Geometry: final body of the model. Coordinates: model frame, mm. A direction names the side the tool comes from. Coordinates: 2 decimals unless noted, no trailing zeros. Order: outer loops, then holes, each group sorted by start corner. A loop starts at its lowest first (then second) coordinate and runs counter-clockwise, first axis right, second up. Notation, with made-up numbers: (-19.75, -11.75) -> (13.25, -11.75) arc R14 cw to (13.25, 8.25) -> close; hole circle Ø1 at (-18.5, -26.5). An arc over 180 degrees is marked (long way). Answer in a Markdown table with one row per item. Add a question column.
1) Ray query, line 1 (Y direction, x = -302, z = -784); line 2 (Z direction, x = -180, y = -136). Return the intervals inside material, ascending. Write a range as from..to.
2) Contact query for flat-ended pins moving along their axis: P1, Ø1.5, axis at x = -223.5, z = -242, coming from the -Y side; P2, Ø4, axis at y = -2, z = -550, coming from the -X side; P3, Ø2, axis at x = -126.5, z = -216, coming from the +Y side. Output: stop coordinate, or through.
3) Section query C-C on z = -466. Return the cut outline in (x, y).
4) Section query A-A on x = -193.5. Return the cut outline in (y, z).
5) Section query B-B on y = -115. Return the cut outline in (x, z), then the cut area to 3 significant figures.
6) Set-up query: faces 1 (the face through (-218, -5.08, -430)), 2 (the face through (-219, 0, -439)). Return all of +Z, -Z, +X, -X, +Y, -Y with unobstructed straight access to the full face (end or side cutting, diameter ignored); none if empty.
```python
from build123d import *

# Parameters (mm, degrees)
F0_W     = 429.031141
F0_H     = 871.334374
F1_DEPTH = 5.08
F2_W     = 431.302786
F2_H     = 296.81766
F3_DEPTH = 5.08


with BuildPart() as f1:
    # F0 (on Front) → F1 (new body)
    with BuildSketch(Plane.XZ):
        with Locations((-214.51557, -435.667187)):
            Rectangle(F0_W, F0_H)
    extrude(amount=F1_DEPTH)

    # F2 (on Top) → F3 (join)
    with BuildSketch(Plane.XY):
        with Locations((-215.651393, -148.40883)):
            Rectangle(F2_W, F2_H)
    extrude(amount=F3_DEPTH)


solid = f1.part
```
Result:
| question | item | result |
|---|---|---|
| 1 | line 1 | -5.08..0 |
| 1 | line 2 | 0..5.08 |
| 2 | P1 | y = -5.08 |
| 2 | P2 | x = -429.03 |
| 2 | P3 | y = 0 |
| 3 | outline | (-429.03, -5.08) -> (0, -5.08) -> (0, 0) -> (-429.03, 0) -> close |
| 4 | outline | (-296.82, 0) -> (-5.08, 0) -> (-5.08, -871.33) -> (0, -871.33) -> (0, 5.08) -> (-296.82, 5.08) -> close |
| 5 | outline | (-431.3, 0) -> (0, 0) -> (0, 5.08) -> (-431.3, 5.08) -> close |
| 5 | area | 2,190 mm2 |
| 6 | face 1 | -Z, +X, -X, -Y |
| 6 | face 2 | +Z, -Z, +X, -X, +Y |
